```python
from build123d import *

# Parameters (mm, degrees)
SKETCH1_R           = 1.5
BOSS_EXTRUDE1_DEPTH = 2


with BuildPart() as part:
    # Sketch1 → Boss-Extrude1 (new body)
    with BuildSketch(Plane(origin=(0, 0, 0), x_dir=(1, 0, 0), z_dir=(0, 1, 0))):
        with BuildLine():
            Line((-8, 4), (8, 4))
            ThreePointArc((8, 4), (10.828427125, 2.828427125), (12, 0))
            Line((12, 0), (11.099, -23.51))
            ThreePointArc((11.099, -23.51), (0, -28.41979688), (-11.099, -23.51))
            Line((-11.099, -23.51), (-12, 0))
            ThreePointArc((-12, 0), (-10.828427125, 2.828427125), (-8, 4))
        make_face()
        with Locations((-8, -1.08)):
            Circle(SKETCH1_R, mode=Mode.SUBTRACT)
        with Locations((8, -1.08)):
            Circle(SKETCH1_R, mode=Mode.SUBTRACT)
    extrude(amount=BOSS_EXTRUDE1_DEPTH)


solid = part.part
```
Build history of the part. All positions in model axes, mm. Give positions to 0.01 mm unless a question says otherwise; leave off trailing zeros. Order: outer loops, then holes, each group sorted by start corner. A loop starts at its lowest first (then second) coordinate and runs counter-clockwise, first axis right, second up. Notation, with made-up numbers: M 85,24.5 L 104,24.5 A28 cw 104,46.5 Z; hole C -20.5,0 d9. An arc over 180 degrees is marked long. Write item = value, one per line. Start each with the question number.
(1) Two-plate mould, pull along Z, no slides. Class faces 1 (the cylindrical face through (10.797, 0.986, -2.859)), 2 (the flat face through (0, 2, 12)), 3 (the cylindrical face through (-9.5, 0.99, 1.01)): released by +Z, released by -Z, zero draft, split by the parting line, or undercut.
(2) Slice it at C-C on x = 10.25. Write the cut outline in (y, z), plus the area to 3 significant figures.
(3) Slice it at B-B on z = 1.08. Write the cut outline in (x, y), plus the area to 3 significant figures.
(4) Probe L1, parallel to X at y = 1.1, z = 1.08; L2, parallel to Z at x = 8, y = 0.7; L3, parallel to Z at x = 7, y = 1.7. List the from-to ranges inside material, lowest first. Write a range as [from, to].
(5) Slice it at A-A on y = 0.9. Write the cut outline in (x, z), plus the area to 3 significant figures.
(6) Slice it at D-D on z = 12.5. Write the cut outline in (x, y), plus the area to 3 significant figures.
(7) Pin check, flat tip, straight feed: pin 1 Ø1.8 at (x, z) = (-8, 1.08) entering from -Y. Stop position of the tip, or through.
Responses:
q1.face_1 = released by -Z
q1.face_2 = zero draft
q1.face_3 = undercut
q2.outline = M 0,-3.31 L 2,-3.31 L 2,24.37 L 0,24.37 Z
q2.area = 55.4 mm2
q3.outline = M -11.96,0 L -9.5,0 L -9.5,2 L -11.96,2 Z; M -6.5,0 L 6.5,0 L 6.5,2 L -6.5,2 Z; M 9.5,0 L 11.96,0 L 11.96,2 L 9.5,2 Z
q3.area = 35.8 mm2
q4.L1 = [-11.96, -9.5], [-6.5, 6.5], [9.5, 11.96]
q4.L2 = [-4, -0.42], [2.58, 26.11]
q4.L3 = [-4, -0.04], [2.2, 26.69]
q5.outline = M -12,0 A4 ccw -8,-4 L 8,-4 A4 ccw 12,0 L 11.1,23.51 A15 ccw -11.1,23.51 Z; hole C -8,1.08 d3; hole C 8,1.08 d3
q5.area = 693 mm2
q6.outline = M -11.52,0 L 11.52,0 L 11.52,2 L -11.52,2 Z
q6.area = 46.1 mm2
q7.pin_1 = through
